```python
from build123d import *

# Parameters (mm, degrees)
LENGTH_DEPTH = 170


with BuildPart() as part:
    # Sketch1 → Length (new body)
    with BuildSketch(Plane.XY):
        with BuildLine():
            Line((0, 0), (0, 18.5))
            Line((0, 18.5), (-0.5, 18.5))
            Line((-0.5, 18.5), (-1.5, 16.5))
            Line((-1.5, 16.5), (-1.5, 13.75))
            Line((-1.5, 13.75), (-1.3, 13.75))
            Line((-1.3, 13.75), (-1.3, 11.25))
            Line((-1.3, 11.25), (-1.5, 11.25))
            Line((-1.5, 11.25), (-1.5, 6.75))
            Line((-1.5, 6.75), (-1.3, 6.75))
            Line((-1.3, 6.75), (-1.3, 4.25))
            Line((-1.3, 4.25), (-1.5, 4.25))
            Line((-1.5, 4.25), (-1.5, 1))
            ThreePointArc((-1.5, 1), (-0.767766953, -0.767766953), (1, -1.5))
            Line((1, -1.5), (4.25, -1.5))
            Line((4.25, -1.5), (4.25, -1.3))
            Line((4.25, -1.3), (6.75, -1.3))
            Line((6.75, -1.3), (6.75, -1.5))
            Line((6.75, -1.5), (11.25, -1.5))
            Line((11.25, -1.5), (11.25, -1.3))
            Line((11.25, -1.3), (13.75, -1.3))
            Line((13.75, -1.3), (13.75, -1.5))
            Line((13.75, -1.5), (16.5, -1.5))
            Line((16.5, -1.5), (18.5, -0.5))
            Line((18.5, -0.5), (18.5, 0))
            Line((18.5, 0), (0, 0))
        make_face()
    extrude(amount=LENGTH_DEPTH)


solid = part.part
```
Source: CAD feature listing. Evaluate the final solid. Frame: model axes, mm. A direction names the side the tool comes from. Round coordinates to 2 decimals unless told otherwise and drop trailing zeros. Loops run counter-clockwise (first coordinate to the right, second up) from the corner with the lowest first, then second, coordinate; pieces in that order, holes last. Notation, with made-up numbers: M 28.25,37.5 L 66.25,37.5 A24 ccw 66.25,68.5 Z; hole C -15,62.25 d7. An arc over 180 degrees is marked long. Put each result on its own line as item: value.
(1) First-contact query: pin 1 (2 mm diameter, centred on y = 13, z = 98, fed in from -X); pin 2 (0.8 mm diameter, centred on x = 6, z = 72.5, fed in from -Y); pin 3 (1 mm diameter, centred on x = 2, z = 121.5, fed in from +Y). Flat tips, straight axial feed; report the tip coordinate or a pass-through.
Solutions:
pin 1: x = -1.5
pin 2: y = -1.3
pin 3: y = 0
(2) Ray query, line 1 (Y direction, x = 4, z = 94); line 2 (X direction, y = 5.75, z = 16). Return the intervals inside material, ascending. Write a range as [from, to].
Solutions:
line 1: [-1.5, 0]
line 2: [-1.3, 0]
(3) Access query for faces 1 (the face through (-1.5, 15, 84)), 2 (the face through (9, 0, 84)). Directions: +Z, -Z, +X, -X, +Y, -Y. A direction counts if a zero-diameter tool reaches every point of the face in a straight line with its end or side. Return the directions, or none.
Solutions:
face 1: +Z, -Z, -X, +Y, -Y
face 2: +Z, -Z, +X, +Y
(4) Section A-A, the plane z = 114. Return loops of the section in (x, y).
Solutions:
outline: M -1.5,1 A2.5 ccw 1,-1.5 L 4.25,-1.5 L 4.25,-1.3 L 6.75,-1.3 L 6.75,-1.5 L 11.25,-1.5 L 11.25,-1.3 L 13.75,-1.3 L 13.75,-1.5 L 16.5,-1.5 L 18.5,-0.5 L 18.5,0 L 0,0 L 0,18.5 L -0.5,18.5 L -1.5,16.5 L -1.5,13.75 L -1.3,13.75 L -1.3,11.25 L -1.5,11.25 L -1.5,6.75 L -1.3,6.75 L -1.3,4.25 L -1.5,4.25 Z
(5) Section B-B, the plane y = 9.5. Return loops of the section in (x, z).
Solutions:
outline: M -1.5,0 L 0,0 L 0,170 L -1.5,170 Z
